Work out the finished part from the listing and answer in its coordinate system (mm). A direction names the side the tool comes from. Round coordinates to 2 decimals unless told otherwise and drop trailing zeros. Order: outer loops, then holes, each group sorted by start corner. A loop starts at its lowest first (then second) coordinate and runs counter-clockwise, first axis right, second up. Notation, with made-up numbers: M -6.5,12.25 L 39.5,12.25 A21 cw 39.5,39.25 Z; hole C 11.5,65.5 d11. An arc over 180 degrees is marked long. Answer as a JSON object with one key per item and string values. Group by question number.
from build123d import *

# Parameters (mm, degrees)
F0_W         = 12.7
F0_H         = 12.7
F0_R         = 9.525
F1_DEPTH     = 25.4
F2_DEPTH     = 38.1
F3_SIZE      = 6.34999
F4_T1_DEPTH  = 50.8
F4_T3_DEPTH  = 99.6409143921
F4_T5_DEPTH  = 25.4
F4_T7_DEPTH  = 45.0011313289
F4_T10_ANGLE = 153.1514920802
F4_T12_ANGLE = 116.8485079198
F5_R         = 6.35
F6_DEPTH     = 50.8010001


# Not quite as in the source:
# - a fillet or chamfer that OpenCascade refuses, or shapes differently, is made with other operations: its cross-section is extruded or revolved along the edge and cut away or added
# - a fillet or chamfer is up to 0.001 mm smaller than in the source, because OpenCascade refuses the exact size


with BuildPart() as f1:
    # F0 (on Top) → F1 (new body)
    with BuildSketch(Plane.XY):
        with Locations((-38.2198102176, 35.4162262917)):
            Rectangle(F0_W, F0_H)
        with BuildLine():
            Line((-6.4698102176, 41.7662262917), (-31.8698102176, 41.7662262917))
            Line((-31.8698102176, 41.7662262917), (-31.8698102176, 29.0662262917))
            Line((-31.8698102176, 29.0662262917), (-44.5698102176, 29.0662262917))
            Line((-44.5698102176, 29.0662262917), (-44.5698102176, -15.9349050373))
            ThreePointArc((-44.5698102176, -15.9349050373), (-31.8698102176, -3.2349050373), (-19.1698102176, -15.9349050373))
            ThreePointArc((-19.1698102176, -15.9349050373), (-21.0500621459, -22.5849465157), (-26.1340703224, -27.2658929842))
            Line((-26.1340703224, -27.2658929842), (62.7659296776, 17.7352383447))
            ThreePointArc((62.7659296776, 17.7352383447), (69.3831964392, 32.0146540993), (57.0301897824, 41.7662262917))
            Line((57.0301897824, 41.7662262917), (6.2301897824, 41.7662262917))
            Line((6.2301897824, 41.7662262917), (6.2301897824, 60.8162262917))
            Line((6.2301897824, 60.8162262917), (-6.4698102176, 60.8162262917))
            Line((-6.4698102176, 60.8162262917), (-6.4698102176, 41.7662262917))
        make_face()
        with BuildLine():
            ThreePointArc((-19.1698102176, -15.9349050373), (-31.8698102176, -3.2349050373), (-44.5698102176, -15.9349050373))
            ThreePointArc((-44.5698102176, -15.9349050373), (-38.5198516961, -26.754653109), (-26.1340703224, -27.2658929842))
            ThreePointArc((-26.1340703224, -27.2658929842), (-21.0500621459, -22.5849465157), (-19.1698102176, -15.9349050373))
        make_face()
        with Locations((-31.8698102176, -15.9349050373)):
            Circle(F0_R, mode=Mode.SUBTRACT)
    extrude(amount=F1_DEPTH)

    # F0 (on Top) → F2 (join)
    with BuildSketch(Plane.XY):
        with Locations((-38.2198102176, 35.4162262917)):
            Rectangle(F0_W, F0_H)
    extrude(amount=F2_DEPTH)

    # F3 (size 6.35 in the source; OpenCascade refuses exactly that, so slightly less here)
    f3_edges = [f1.edges().sort_by_distance(p)[0] for p in [
        (-38.21981, 29.066226, 38.1),
        (-44.56981, 35.416226, 38.1),
        (-38.21981, 41.766226, 38.1),
        (-31.86981, 35.416226, 38.1),
    ]]
    chamfer(f3_edges, length=F3_SIZE)

    # F4: fillet of radius 12.7 on 6 edges, made by hand

    # F4_s2 → F4_t1 (cut)
    with BuildSketch(Plane.YZ.offset(6.2301897824)):
        with BuildLine():
            ThreePointArc((29.0662262917, 25.4), (38.0464824127, 21.6802561211), (41.7662262917, 12.7))
            Line((41.7662262917, 12.7), (42.0202262917, 12.7))
            Line((42.0202262917, 12.7), (42.0202262917, 25.654))
            Line((42.0202262917, 25.654), (29.0662262917, 25.654))
            Line((29.0662262917, 25.654), (29.0662262917, 25.4))
        make_face()
    extrude(amount=F4_T1_DEPTH, mode=Mode.SUBTRACT)

    # F4_s4 → F4_t3 (cut)
    with BuildSketch(Plane(origin=(-31.7901974435, -16.0921805414, 0), x_dir=(0, 0, 1), z_dir=(0.8922037754, 0.4516330626, 0))):
        with BuildLine():
            ThreePointArc((25.4, -0.1762775595), (21.6802561211, 8.8039785616), (12.7, 12.5237224405))
            Line((12.7, 12.5237224405), (12.7, 12.7777224405))
            Line((12.7, 12.7777224405), (25.654, 12.7777224405))
            Line((25.654, 12.7777224405), (25.654, -0.1762775595))
            Line((25.654, -0.1762775595), (25.4, -0.1762775595))
        make_face()
    extrude(amount=F4_T3_DEPTH, mode=Mode.SUBTRACT)

    # F4_s6 → F4_t5 (cut)
    with BuildSketch(Plane.YZ.offset(-31.8698102176)):
        with BuildLine():
            ThreePointArc((41.7662262917, 12.7), (38.0464824127, 21.6802561211), (29.0662262917, 25.4))
            Line((29.0662262917, 25.4), (29.0662262917, 25.654))
            Line((29.0662262917, 25.654), (42.0202262917, 25.654))
            Line((42.0202262917, 25.654), (42.0202262917, 12.7))
            Line((42.0202262917, 12.7), (41.7662262917, 12.7))
        make_face()
    extrude(amount=F4_T5_DEPTH, mode=Mode.SUBTRACT)

    # F4_s8 → F4_t7 (cut)
    with BuildSketch(Plane.XZ.offset(-29.0662262917)):
        with BuildLine():
            ThreePointArc((-44.5698102176, 12.7), (-40.8500663387, 21.6802561211), (-31.8698102176, 25.4))
            Line((-31.8698102176, 25.4), (-31.8698102176, 25.654))
            Line((-31.8698102176, 25.654), (-44.8238102176, 25.654))
            Line((-44.8238102176, 25.654), (-44.8238102176, 12.7))
            Line((-44.8238102176, 12.7), (-44.5698102176, 12.7))
        make_face()
    extrude(amount=F4_T7_DEPTH, mode=Mode.SUBTRACT)

    # F4_s9 → F4_t10 (revolve, cut)
    with BuildSketch(Plane(origin=(57.1098025565, 28.9089507875, 0), x_dir=(0, 0, 1), z_dir=(-0.8922037754, -0.4516330626, 0))):
        with BuildLine():
            ThreePointArc((25.4, 0.1762775595), (21.6802561211, -8.8039785616), (12.7, -12.5237224405))
            Line((12.7, -12.5237224405), (12.7, -12.7777224405))
            Line((12.7, -12.7777224405), (25.654, -12.7777224405))
            Line((25.654, -12.7777224405), (25.654, 0.1762775595))
            Line((25.654, 0.1762775595), (25.4, 0.1762775595))
        make_face()
    revolve(axis=Axis((57.0301897824, 29.0662262917, 25.4), (0, 0, 1)), revolution_arc=F4_T10_ANGLE, mode=Mode.SUBTRACT)

    # F4_s11 → F4_t12 (revolve, cut)
    with BuildSketch(Plane.XZ.offset(15.9349050373)):
        with BuildLine():
            ThreePointArc((-44.5698102176, 12.7), (-40.8500663387, 21.6802561211), (-31.8698102176, 25.4))
            Line((-31.8698102176, 25.4), (-31.8698102176, 25.654))
            Line((-31.8698102176, 25.654), (-44.8238102176, 25.654))
            Line((-44.8238102176, 25.654), (-44.8238102176, 12.7))
            Line((-44.8238102176, 12.7), (-44.5698102176, 12.7))
        make_face()
    revolve(axis=Axis((-31.8698102176, -15.9349050373, 25.4), (0, 0, 1)), revolution_arc=F4_T12_ANGLE, mode=Mode.SUBTRACT)

    # F5 (on face) → F6 (cut, through all)
    with BuildSketch(Plane.YZ.offset(6.2301897824)):
        with Locations((51.2912262917, 12.7)):
            Circle(F5_R)
    extrude(amount=-F6_DEPTH, mode=Mode.SUBTRACT)


solid = f1.part
Item 1: Find section B-B (y = 33). Give the vertices of the cut face in (x, z).
Item 2: Find section A-A (z = 27). Give the vertices of the cut face in (x, y).
Item 3: Consider L1, parallel to X at y = 33.5, z = 29.5; L2, parallel to X at y = -24.5, z = 6; L3, parallel to Z at x = 20, y = 20. Determine where each line is inside the solid, lowest interval first.
Item 4: A tool of negligible diameter and unlimited length cuts with its end or side. For faces 4 (the flat face through (-31.87, 37, 26)), 5 (the flat face through (32, 41.766, 6)), 6 (the flat face through (-29, 41.766, 12)), from which of +Z, -Z, +X, -X, +Y, -Y can it reach the whole face along a straight path? Write none if from no direction.
Item 5: Each of these flat-tipped pins is pushed along its axis until it touches: pin 1 (12 mm diameter, centred on y = 52, z = 19.5, fed in from +X); pin 2 (5 mm diameter, centred on x = -14, z = 24.5, fed in from +Y); pin 3 (1 mm diameter, centred on x = 16, y = -3.5, fed in from +Z). Where does it stop, or does it pass through?
Item 6: The mould has two halves that part along Y. Classify faces 1 (the cylindrical face through (-0.031, 57.348, 14.607)), 2 (the cylindrical face through (-19.348, 38.145, 21.581)), 3 (the cylindrical face through (-38.67, -26.66, 6.26)): +Y half, -Y half, draft (parallel to the pull), parting line (faces both ways), or undercut.
Responses:
{
 "1": {"outline": "M -44.57,0 L 69.11,0 L 69.11,12.7 A12.08 ccw 57.03,24.78 L 6.23,24.78 L 6.23,25.4 L -6.47,25.4 L -6.47,24.78 L -31.87,24.78 L -31.87,31.75 L -35.8,35.68 L -40.64,35.68 L -44.57,31.75 Z"},
 "2": {"outline": "M -44.57,29.07 L -31.87,29.07 L -31.87,41.77 L -44.57,41.77 Z"},
 "3": {"L1": "x = -44.57 to -31.87", "L2": "x = -41.25 to -36.04, -27.7 to -20.67", "L3": "z = 0 to 25.4"},
 "4": {"face 4": "+Z, +Y", "face 5": "+Z, -Z, +X, +Y", "face 6": "+Z, -Z, -X, +Y"},
 "5": {"pin 1": "stops at x = 6.23", "pin 2": "stops at y = 37.71", "pin 3": "stops at z = 20.5"},
 "6": {"face 1": "undercut", "face 2": "+Y half", "face 3": "-Y half"}
}
